Answer from the drawing. Dimensions are ordinates in mm from the lowest x, y and z of the part. A direction names the side the tool comes from. Coordinates: 2 decimals unless noted, no trailing zeros. Write each loop counter-clockwise with the first axis right and the second up, starting at its lowest first coordinate (ties: lowest second). Pieces come first, ordered by that corner, then holes.
(1) Given pin 1 (22.5 mm diameter, centred on x = 15.5, z = 32.5, fed in from +Y); pin 2 (5 mm diameter, centred on y = 11.5, z = 36.5, fed in from -X), each flat-ended and moving along its own axis, determine where each tip first touches the part or whether it passes through.
(2) Section D-D on z = 15 is taken. Write down the section's boundary in (x, y).
(3) Section B-B on x = 38 is taken. Write down the section's boundary in (y, z).
(4) Find the intervals of material crossed by probe 1 along Z at (x, y) = (12, 2.2); probe 2 along X at (y, z) = (1, 6); probe 3 along Y at (x, z) = (51, 40), in increasing order.
(5) Section C-C on y = 44 is taken. Write down the section's boundary in (x, z).
(6) Which of the six approach directions +Z, -Z, +X, -X, +Y, -Y give full straight-line access (tool end or side, diameter ignored) to the marked faces 1 and 2?
(7) Section A-A on z = 22.5 is taken. Write down the section's boundary in (x, y).
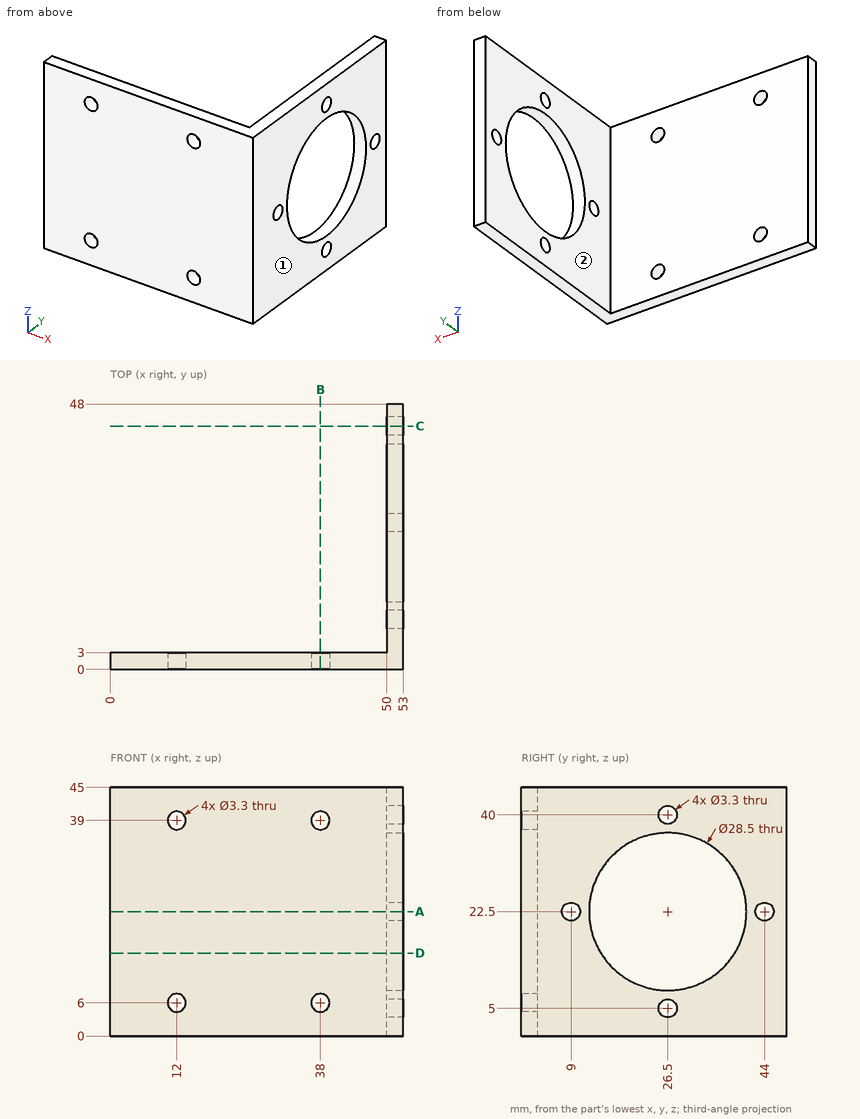
Response:
1. pin 1: stops at y = 3
1. pin 2: stops at x = 50
2. outline: (0, 0) - (53, 0) - (53, 14.38) - (50, 14.38) - (50, 3) - (0, 3) - close; (50, 38.62) - (53, 38.62) - (53, 48) - (50, 48) - close
3. outline: (0, 0) - (3, 0) - (3, 4.35) - (0, 4.35) - close; (0, 7.65) - (3, 7.65) - (3, 37.35) - (0, 37.35) - close; (0, 40.65) - (3, 40.65) - (3, 45) - (0, 45) - close
4. probe 1: z = 0 to 4.35, 7.65 to 37.35, 40.65 to 45
4. probe 2: x = 0 to 10.35, 13.65 to 36.35, 39.65 to 53
4. probe 3: y = 0 to 24.85, 28.15 to 48
5. outline: (50, 0) - (53, 0) - (53, 20.85) - (50, 20.85) - close; (50, 24.15) - (53, 24.15) - (53, 45) - (50, 45) - close
6. face 1: +Z, -Z, +X, +Y, -Y
6. face 2: +Z, -Z, -X, +Y
7. outline: (0, 0) - (53, 0) - (53, 7.35) - (50, 7.35) - (50, 3) - (0, 3) - close; (50, 10.65) - (53, 10.65) - (53, 12.25) - (50, 12.25) - close; (50, 40.75) - (53, 40.75) - (53, 42.35) - (50, 42.35) - close; (50, 45.65) - (53, 45.65) - (53, 48) - (50, 48) - close
